The model under review builds one solid part; all positions refer to its coordinate system, in mm. Face numbers are marked on the shaded views. Give positions to 0.01 mm unless a question says otherwise; leave off trailing zeros. Order: outer loops, then holes, each group sorted by start corner. A loop starts at its lowest first (then second) coordinate and runs counter-clockwise, first axis right, second up. Notation, with made-up numbers: (-36.75, 2.25) -> (-3.75, 2.25) arc R15 cw to (-3.75, 9.25) -> close; hole circle Ø3 at (-25, -12). An arc over 180 degrees is marked (long way). Answer as a JSON object with one key per item and string values. Group by question number.
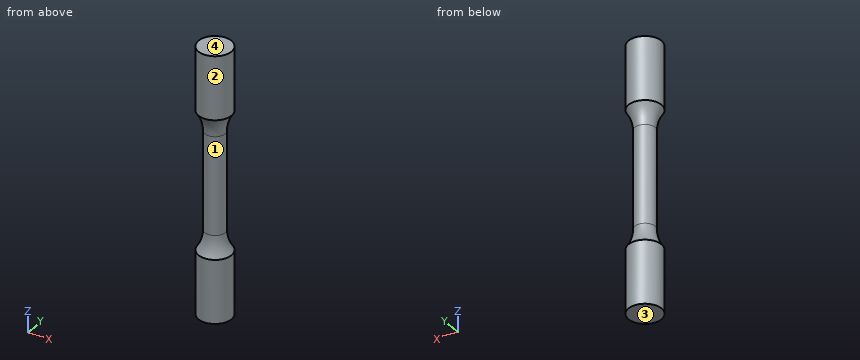
from build123d import *

# Parameters (mm, degrees)
F0_W = 7.5
F0_H = 120


with BuildPart() as f1:
    # F0 (on Front) → F1 (revolve)
    with BuildSketch(Plane.XZ):
        with Locations((3.75, 60)):
            Rectangle(F0_W, F0_H)
    revolve(axis=Axis((0, 0, 60), (0, 0, 1)))

    # F2 (on Front) → F3 (revolve, cut)
    with BuildSketch(Plane.XZ):
        with BuildLine():
            ThreePointArc((-20.40513, 22.038545), (-9.22552, 26.669291), (-4.594774, 37.848901))
            Line((-4.594774, 37.848901), (-4.594774, 82.151099))
            ThreePointArc((-4.594774, 82.151099), (-9.22552, 93.330709), (-20.40513, 97.961455))
            Line((-20.40513, 97.961455), (-20.40513, 22.038545))
        make_face()
    revolve(axis=Axis((0, 0, 57.177005), (0, 0, 1)), mode=Mode.SUBTRACT)


solid = f1.part
1. Take a section at A-A on x = 0. Give the boundary of the cut face in (y, z).
2. Take a section at D-D on z = 60.5. Give the boundary of the cut face in (x, y), plus the area to 3 significant figures.
3. Draft analysis for pull direction Z (two halves, no side actions). For the marked faces 1, 2, 3 and 4, state which applies: pulls with the +Z half, pulls with the -Z half, needs draft (parallel to the pull), parting line crosses it, or undercut.
4. Take a section at C-C on z = 106. Give the boundary of the cut face in (x, y).
5. For pin 1 (3 mm diameter, centred on x = -5, z = 105.5, fed in from -Y); pin 2 (1 mm diameter, centred on y = -5.5, z = 15, fed in from +X); pin 3 (1 mm diameter, centred on x = -1.5, z = 98.5, fed in from +Y), all flat-tipped, find the tip position at first contact; note any pin that passes through.
6. For probe 1 along Y at (x, z) = (-0.25, 97); probe 2 along Z at (x, y) = (7.25, -1.75); probe 3 along Z at (x, y) = (-4, -5.5), list the stretches that pass through material, from the lowest coordinate up. Write a range as [from, to].
Checks:
{
 "1": {"outline": "(-7.5, 0) -> (7.5, 0) -> (7.5, 28.72) arc R15.81 cw to (4.59, 37.85) -> (4.59, 82.15) arc R15.81 cw to (7.5, 91.28) -> (7.5, 120) -> (-7.5, 120) -> (-7.5, 91.28) arc R15.81 cw to (-4.59, 82.15) -> (-4.59, 37.85) arc R15.81 cw to (-7.5, 28.72) -> close"},
 "2": {"outline": "circle Ø9.19 at (0, 0)", "area": "66.3 mm2"},
 "3": {"face 1": "undercut", "face 2": "needs draft", "face 3": "pulls with the -Z half", "face 4": "pulls with the +Z half"},
 "4": {"outline": "circle Ø15 at (0, 0)"},
 "5": {"pin 1": "stops at y = -6.63", "pin 2": "stops at x = 5.59", "pin 3": "stops at y = 7.43"},
 "6": {"probe 1": "y = [-7.5, 7.5]", "probe 2": "z = [0, 28.77], [91.23, 120]", "probe 3": "z = [0, 29.79], [90.21, 120]"}
}
